Could you check a few things on this drawing? It's one solid part, dimensions in mm from its lowest x, y, z. Give positions to 0.01 mm unless a question says otherwise; leave off trailing zeros. Order: outer loops, then holes, each group sorted by start corner. A loop starts at its lowest first (then second) coordinate and runs counter-clockwise, first axis right, second up.
Item 1: I want a section at A-A, the plane x = 52. Write out the boundary of the cut face in (y, z).
Item 2: I want a section at B-B, the plane y = 46.5. Write out the boundary of the cut face in (x, z), then the cut area to 3 significant figures.
Item 3: I want a section at C-C, the plane z = 1.85. Write out the boundary of the cut face in (x, y).
Item 4: If I drill on line 1 along Y through (x, z) = (3, 0.4); line 2 along X through (y, z) = (39.5, 2.4), over which ranges is the centre line in solid material (lowest first)?
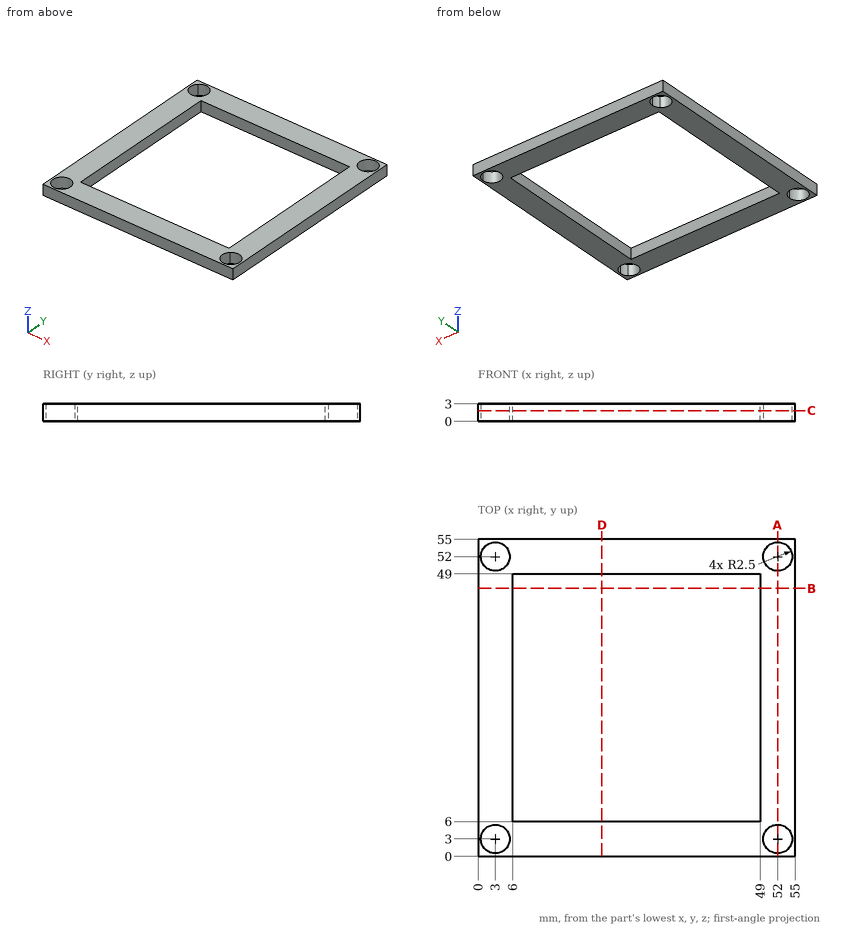
Results list:
1. outline: (0, 0) - (0.5, 0) - (0.5, 3) - (0, 3) - close; (5.5, 0) - (49.5, 0) - (49.5, 3) - (5.5, 3) - close; (54.5, 0) - (55, 0) - (55, 3) - (54.5, 3) - close
2. outline: (0, 0) - (6, 0) - (6, 3) - (0, 3) - close; (49, 0) - (55, 0) - (55, 3) - (49, 3) - close
2. area: 36.0 mm2
3. outline: (0, 0) - (55, 0) - (55, 55) - (0, 55) - close; hole (4.77, 4.77) arc R2.5 ccw (long way) to (5.5, 3) arc R2.5 ccw to start; hole (4.77, 50.23) arc R2.5 ccw to (5.5, 52) arc R2.5 ccw (long way) to start; hole (6, 6) - (49, 6) - (49, 49) - (6, 49) - close; hole (53.77, 1.23) arc R2.5 ccw to (54.5, 3) arc R2.5 ccw (long way) to start; hole (53.77, 53.77) arc R2.5 ccw (long way) to (54.5, 52) arc R2.5 ccw to start
4. line 1: y = 0 to 0.5, 5.5 to 49.5, 54.5 to 55
4. line 2: x = 0 to 6, 49 to 55
